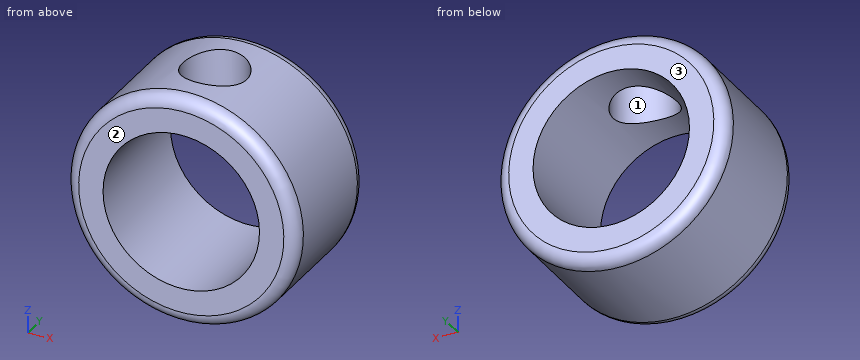
```python
from build123d import *

# Parameters (mm, degrees)
SKETCH1_R                  = 4.5
BOSS_EXTRUDE1_DEPTH        = 5
F_6_1_6_1_DIAMETER_HOLE1_D = 6.1
SKETCH6_W                  = 1.25
SKETCH6_H                  = 4.5
FILLET1_R                  = 0.5


with BuildPart() as part:
    # Sketch1 → Boss-Extrude1 (new body)
    with BuildSketch(Plane(origin=(0, 0, 0), x_dir=(1, 0, 0), z_dir=(0, 1, 0))):
        with Locations(Location((0, 0, 0), (0, 0, 270))):
            Circle(SKETCH1_R)
    extrude(amount=BOSS_EXTRUDE1_DEPTH)

    # Ø6.1 (6.1) Diameter Hole1 (through all)
    with Locations(Plane(origin=(0, 5, 0), x_dir=(1, 0, 0), z_dir=(0, 1, 0))):
        with Locations((0, 0)):
            Hole(F_6_1_6_1_DIAMETER_HOLE1_D / 2)

    # Sketch6 → M3 Tapped Hole1 (revolve, cut)
    with BuildSketch(Plane(origin=(-0.007135696, 2.5, 0), x_dir=(0, 1, 0), z_dir=(1, 0, 0))):
        with Locations((0.625, 2.25)):
            Rectangle(SKETCH6_W, SKETCH6_H)
    revolve(axis=Axis((-0.007135696, 2.5, -6.35), (0, 0, 1)), mode=Mode.SUBTRACT)

    # Fillet1
    fillet1_edges = [part.edges().sort_by_distance(p)[0] for p in [
        (0, 0, -4.5),
        (0, 5, -4.5),
    ]]
    fillet(fillet1_edges, radius=FILLET1_R)


solid = part.part
```
CAD build for the part. Positions are in the model's coordinates, mm. Face numbers are marked on the shaded views. Coordinates: 2 decimals unless noted, no trailing zeros. Order: outer loops, then holes, each group sorted by start corner. A loop starts at its lowest first (then second) coordinate and runs counter-clockwise, first axis right, second up. Notation, with made-up numbers: (13.25, 80) - (25.25, 80) arc R7 ccw to (25.25, 92) - close; hole circle Ø1 at (56, -26). An arc over 180 degrees is marked (long way). Answer in a Markdown table with one row per item.
1. Slice it at D-D, the plane y = 2. List the corners of the cut face in (x, z), then the cut area to 3 significant figures.
Answer:
| item | result |
|---|---|
| outline | (-1.15, 2.82) - (-1.15, 4.35) arc R4.5 ccw (long way) to (1.14, 4.35) - (1.14, 2.83) arc R3.05 cw (long way) to start |
| area | 31.0 mm² |
2. Slice it at C-C, the plane x = 0.25. Give the number of separate pieces and of enclosed holes in the cut face, then the cut area to 3 significant figures.
Answer:
| item | result |
|---|---|
| separate pieces | 3 |
| enclosed holes | 0 |
| area | 10.8 mm² |
3. Slice it at A-A, the plane z = 0. List the corners of the cut face in (x, y).
Answer:
| item | result |
|---|---|
| outline | (-4.5, 0.5) arc R0.5 ccw to (-4, 0) - (-3.05, 0) - (-3.05, 5) - (-4, 5) arc R0.5 ccw to (-4.5, 4.5) - close; (3.05, 0) - (4, 0) arc R0.5 ccw to (4.5, 0.5) - (4.5, 4.5) arc R0.5 ccw to (4, 5) - (3.05, 5) - close |
4. Drill centre lines: L1, parallel to X at y = 3.9, z = 0.25; L2, parallel to X at y = 2.5, z = 3.2; L3, parallel to Z at x = 1.75, y = 1.45. Where is each one in solid material? Low to high. Write a range as from..to.
Answer:
| item | result |
|---|---|
| L1 | -4.49..-3.04, 3.04..4.49 |
| L2 | -3.16..-1.26, 1.24..3.16 |
| L3 | -4.15..-2.5, 2.5..4.15 |
5. Slice it at B-B, the plane y = 0.7. List the corners of the cut face in (x, z), then the cut area to 3 significant figures.
Answer:
| item | result |
|---|---|
| outline | circle Ø9 at (0, 0); hole circle Ø6.1 at (0, 0) |
| area | 34.4 mm² |
6. Pull direction Y, two halves, no side cores. Call the marked faces 1, 2 and 3: +Y half, -Y half, draft (parallel to the pull), parting line (faces both ways), or undercut.
Answer:
| item | result |
|---|---|
| face 1 | undercut |
| face 2 | -Y half |
| face 3 | +Y half |
7. Flat gauge pins, fed straight in: P1, Ø2, axis at y = 2.5, z = 3, coming from the -X side; P2, Ø2, axis at x = -0.01, y = 2.5, coming from the +Z side. Where does each tip first touch, or does it go through?
Answer:
| item | result |
|---|---|
| P1 | x = -4.03 |
| P2 | z = -2.88 |
